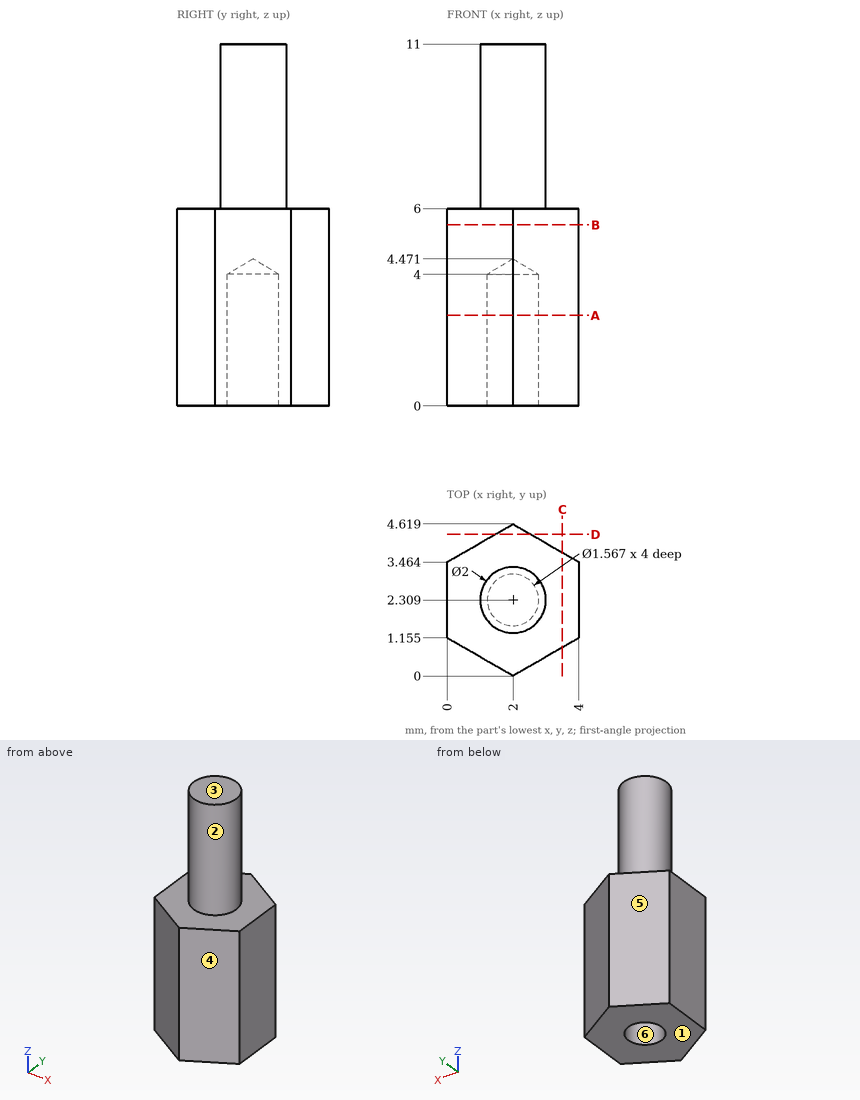
Can you work these out from the drawing? Everything is in mm from the part's minimum corner. A direction names the side the tool comes from. Round coordinates to 2 decimals unless told otherwise and drop trailing zeros. Write each loop counter-clockwise with the first axis right and the second up, starting at its lowest first coordinate (ties: lowest second). Pieces come first, ordered by that corner, then holes. Notation, with made-up numbers: M 87,39.5 L 109,39.5 A17 ccw 109,65.5 Z; hole C -7,84.5 d4. An arc over 180 degrees is marked long. Use a Markdown table: item, result.
Item 1: I want a section at D-D (y = 4.3). List the corners of the cut face in (x, z) for me.
Found:
| item | result |
|---|---|
| outline | M 1.45,0 L 2.55,0 L 2.55,6 L 1.45,6 Z |
Item 2: I want a section at A-A (z = 2.75). List the corners of the cut face in (x, y) for me (1 decimal).
Found:
| item | result |
|---|---|
| outline | M 0,1.2 L 2,0 L 4,1.2 L 4,3.5 L 2,4.6 L 0,3.5 Z; hole C 2,2.3 d1.6 |
Item 3: We'd pull the mould along Y, two halves only. Please class the marked faces 3, 4, 5 and 6: released by +Y, released by -Y, zero draft, split by the parting line, or undercut.
Found:
| item | result |
|---|---|
| face 3 | zero draft |
| face 4 | released by -Y |
| face 5 | released by +Y |
| face 6 | undercut |
Item 4: Which directions (+Z, -Z, +X, -X, +Y, -Y) give clear straight access to the entire face, cutting with the end or side of a thin tool? Please do the marked faces 1 and 2.
Found:
| item | result |
|---|---|
| face 1 | -Z, +X, -X, +Y, -Y |
| face 2 | +Z |
Item 5: I want a section at C-C (x = 3.5). List the corners of the cut face in (y, z) for me.
Found:
| item | result |
|---|---|
| outline | M 0.87,0 L 3.75,0 L 3.75,6 L 0.87,6 Z |
Item 6: I want a section at B-B (z = 5.5). List the corners of the cut face in (x, y) for me (1 decimal).
Found:
| item | result |
|---|---|
| outline | M 0,1.2 L 2,0 L 4,1.2 L 4,3.5 L 2,4.6 L 0,3.5 Z |
Item 7: If I drill on line 1 along Z through (x, y) = (2.75, 0.7); line 2 along X through (y, z) = (2.3, 0.5); line 3 along Y through (x, z) = (1.75, 2.75) (1 decimal), over which ranges is the centre line in solid material (lowest first)? Write a range as [from, to].
Found:
| item | result |
|---|---|
| line 1 | z = [0, 6] |
| line 2 | x = [0, 1.22], [2.78, 4] |
| line 3 | y = [0.1, 1.6], [3.1, 4.5] |
